The listing builds one solid part. Answer for the finished solid, in the listing's coordinates (mm). Round coordinates to 2 decimals unless told otherwise and drop trailing zeros. Loops run counter-clockwise (first coordinate to the right, second up) from the corner with the lowest first, then second, coordinate; pieces in that order, holes last. Notation, with made-up numbers: (-18, 20) -> (26, 20) arc R34 cw to (26, 55) -> close; hole circle Ø10 at (62.5, 3). An arc over 180 degrees is marked (long way). Write each question's results on one line, items separated by ' | '. Start each with the question number.
(1) The part is cut by section A-A (x = 75). Determine the outline of the cut face in (y, z), plus the area to 3 significant figures.
(2) Straight lines are drawn through the part: probe 1 along Y at (x, z) = (75, 3.25); probe 2 along Y at (x, z) = (77.5, 4.5); probe 3 along X at (y, z) = (79.5, 11.25). For each, find the intervals that lie inside material, in ascending order.
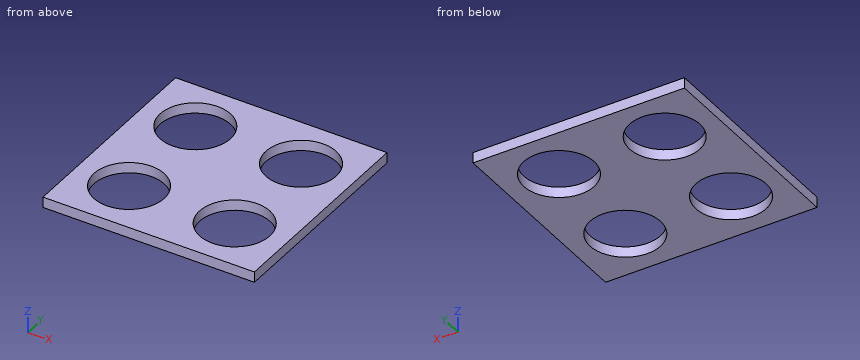
Autodesk Inventor part; units mm, degrees
ref_plane "YZ Plane" through (0, 0, 0) normal (1, 0, 0) x (0, 1, 0)
ref_plane "XZ Plane" through (0, 0, 0) normal (0, 1, 0) x (-1, 0, 0)
ref_plane "XY Plane" through (0, 0, 0) normal (0, 0, 1) x (1, 0, 0)
sketch "スケッチ1" plane through (0, 0, 0) normal (0, 0, 1) x (1, 0, 0)
  line L0 (-150, 150) -> (150, 150)
  line L1 (150, 150) -> (150, -150)
  line L2 (150, -150) -> (-150, -150)
  line L3 (-150, -150) -> (-150, 150)
  circle A0 centre (-75, 75) radius 50
  circle A1 centre (-75, -75) radius 50
  circle A2 centre (75, -75) radius 50
  circle A3 centre (75, 75) radius 50
  point P0 (0, 0)
  point P1 (0, 0)
  dimension "d0" = 300
  dimension "d1" = 100
  dimension "d2" = 100
  dimension "d3" = 100
  dimension "d4" = 100
  dimension "d5" = 150
  dimension "d6" = 150
  dimension "d7" = 75
  dimension "d8" = 75
extrude "押し出し1" add sketch "スケッチ1" along normal blind 15
sketch "スケッチ2" plane through (0, 0, 15) normal (0, 0, 1) x (1, 0, 0)
  circle A0 centre (0, 0) radius 0.005
  dimension "d11" = 0.01
extrude "押し出し2" cut sketch "スケッチ2" against normal through all
properties part number "障害物、丸４"
Checked values:
1) outline: (-150, 0) -> (-125, 0) -> (-125, 15) -> (-150, 15) -> close; (-25, 0) -> (25, 0) -> (25, 15) -> (-25, 15) -> close; (125, 0) -> (150, 0) -> (150, 15) -> (125, 15) -> close | area: 1,500 mm2
2) probe 1: y = -150 to -125, -25 to 25, 125 to 150 | probe 2: y = -150 to -124.94, -25.06 to 25.06, 124.94 to 150 | probe 3: x = -150 to -124.8, -25.2 to 25.2, 124.8 to 150
